CAD build for the part. Positions are in the model's coordinates, mm. Face numbers are marked on the shaded views. A direction names the side the tool comes from. Round coordinates to 2 decimals unless told otherwise and drop trailing zeros. Loops run counter-clockwise (first coordinate to the right, second up) from the corner with the lowest first, then second, coordinate; pieces in that order, holes last.
```python
from build123d import *

# Parameters (mm, degrees)
BASPROSKE_W        = 3
BASPROSKE_H        = 11
TOOTHCUT_DEPTH     = 16.842979518
TEETHCUTS_COUNT    = 20
TEETHCUTS_ANGLE    = 342
BORSKE_R           = 1.5
BORE_DEPTH         = 50.0000508
SKETCH1_R          = 2
CUT_EXTRUDE1_DEPTH = 16.706934942


with BuildPart() as part:
    # BasProSke → Base-Revolve (revolve)
    with BuildSketch(Plane(origin=(0, 0, 0), x_dir=(1, 0, 0), z_dir=(0, 1, 0)), mode=Mode.PRIVATE) as base_revolve_sk:
        with Locations((1.5, 5.5)):
            Rectangle(BASPROSKE_W, BASPROSKE_H)
    revolve(base_revolve_sk.sketch.rotate(Axis((-10, 0, 0), (1, 0, 0)), 180), axis=Axis((-10, 0, 0), (1, 0, 0)))

    # TooCutSke → ToothCut (cut, through all)
    with BuildSketch(Plane(origin=(0, 0, 0), x_dir=(0, 0, -1), z_dir=(1, 0, 0))):
        with BuildLine():
            ThreePointArc((0.499924007, 8.734705318), (0, 8.749), (-0.499924007, 8.734705318))
            ThreePointArc((-0.499924007, 8.734705318), (-0.824302243, 9.905497836), (-1.485192705, 10.924909509))
            ThreePointArc((-1.485192705, 10.924909509), (0, 11.0254), (1.485192705, 10.924909509))
            ThreePointArc((1.485192705, 10.924909509), (0.824302243, 9.905497836), (0.499924007, 8.734705318))
        make_face()
    toothcut = extrude(amount=TOOTHCUT_DEPTH, mode=Mode.SUBTRACT)

    # TeethCuts: ToothCut ×20 about axis
    teethcuts_axis = Axis((-10, 0, 0), (1, 0, 0))
    for i in range(1, TEETHCUTS_COUNT):
        add(toothcut.rotate(teethcuts_axis, i * TEETHCUTS_ANGLE / (TEETHCUTS_COUNT - 1)), mode=Mode.SUBTRACT)

    # BorSke → Bore (cut, symmetric)
    with BuildSketch(Plane(origin=(0, 0, 0), x_dir=(0, 0, -1), z_dir=(1, 0, 0))):
        with Locations(Location((0, 0, 0), (0, 0, 180))):
            Circle(BORSKE_R)
    extrude(amount=BORE_DEPTH, both=True, mode=Mode.SUBTRACT)

    # Sketch1 → Cut-Extrude1 (cut, through all)
    with BuildSketch(Plane(origin=(3, 0, 0), x_dir=(0, 0, -1), z_dir=(1, 0, 0))):
        Circle(SKETCH1_R)
    extrude(amount=-CUT_EXTRUDE1_DEPTH, mode=Mode.SUBTRACT)


solid = part.part
```
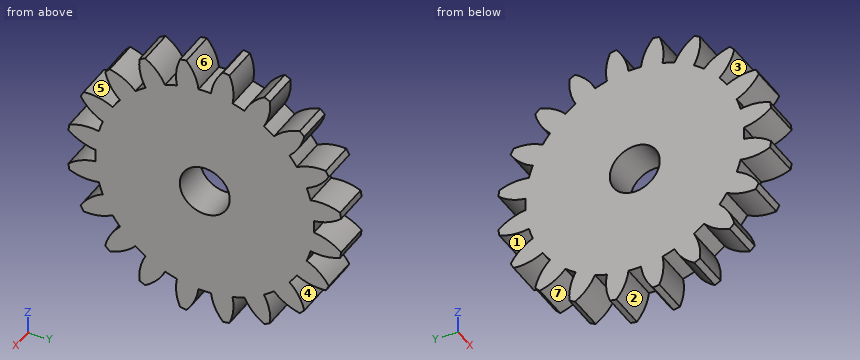
Item 1: Cut at A-A, the plane y = 0. Give the cut face in (x, z).
Answers follow:
outline: (0, -8.75) - (3, -8.75) - (3, -2) - (0, -2) - close; (0, 2) - (3, 2) - (3, 8.75) - (0, 8.75) - close
Item 2: 3-axis set-ups, long thin cutter, end or side, ignore diameter. For the marked faces 1, 2, 3 and 4: which of +Z, -Z, +X, -X, +Y, -Y reach the whole face in a straight line?
Answers follow:
face 1: +X, -X
face 2: -Z, +X, -X
face 3: +X, -X, -Y
face 4: +X, -X, +Y
Item 3: Two-plate mould, pull along Z, no slides. Class the marked faces 5, 6 and 7: released by +Z, released by -Z, zero draft, split by the parting line, or undercut.
Answers follow:
face 5: undercut
face 6: released by +Z
face 7: released by -Z
Item 4: Cut at C-C, the plane z = -3.5. Give the cut face in (x, y).
Answers follow:
outline: (0, -8.73) - (3, -8.73) - (3, 8.73) - (0, 8.73) - close
Item 5: Flat gauge pin, fed straight in: P1, Ø10, axis at y = 5.5, z = -6, coming from the -X side. Where does the tip first touch, or does it go through?
Answers follow:
P1: stops at x = 0
Item 6: Probe line 1 (Y direction, x = 1.15, z = 0); line 2 (Y direction, x = 0.65, z = -8.5); line 3 (Y direction, x = 0.3, z = 9). List the from-to ranges inside material, lowest first.
Answers follow:
line 1: y = -8.75 to -2, 2 to 8.75
line 2: y = -5.16 to -3.36, -2.23 to 2.23, 3.36 to 5.16
line 3: y = -5.23 to -3.7, -2.29 to -0.54, 0.54 to 2.29, 3.7 to 5.23
Item 7: Cut at D-D, the plane y = 2.75. Give the cut face in (x, z).
Answers follow:
outline: (0, -8.31) - (3, -8.31) - (3, 8.31) - (0, 8.31) - close
